Here's how the part is built. I have some questions about the finished solid (model axes, mm). Face numbers are marked on the shaded views. A direction names the side the tool comes from. Give positions to 0.01 mm unless a question says otherwise; leave off trailing zeros. Write each loop counter-clockwise with the first axis right and the second up, starting at its lowest first coordinate (ties: lowest second). Pieces come first, ordered by that corner, then holes. Notation, with made-up numbers: (70.25, 36.5) -> (79.25, 36.5) arc R14 cw to (79.25, 62.5) -> close; hole circle Ø7 at (89, 35). An arc over 180 degrees is marked (long way). Use one line per item in the form item = value.
```python
from build123d import *

# Parameters (mm, degrees)
F0_W     = 15
F0_H     = 9
F0_W_2   = 11
F0_H_2   = 5
F1_DEPTH = 4
F2_R     = 0.99999


# Not quite as in the source:
# - a fillet or chamfer is up to 0.001 mm smaller than in the source, because OpenCascade refuses the exact size


with BuildPart() as f1:
    # F0 (on Top) → F1 (new body)
    with BuildSketch(Plane.XY):
        with Locations((5.5, 2.5)):
            Rectangle(F0_W, F0_H)
        with Locations((5.5, 2.5)):
            Rectangle(F0_W_2, F0_H_2, mode=Mode.SUBTRACT)
    extrude(amount=F1_DEPTH)

    # F2 (radius 1 in the source; OpenCascade refuses exactly that, so slightly less here)
    f2_edges = [f1.edges().sort_by_distance(p)[0] for p in [
        (5.5, -2, 4),
        (13, 2.5, 4),
        (5.5, 0, 4),
        (-2, 2.5, 4),
        (0, 2.5, 4),
        (5.5, 7, 4),
        (5.5, 5, 4),
        (11, 2.5, 4),
        (-2, -2, 2),
        (13, -2, 2),
        (11, 0, 2),
        (0, 0, 2),
        (-2, 7, 2),
        (13, 7, 2),
        (11, 5, 2),
        (0, 5, 2),
    ]]
    fillet(f2_edges, radius=F2_R)


solid = f1.part
```
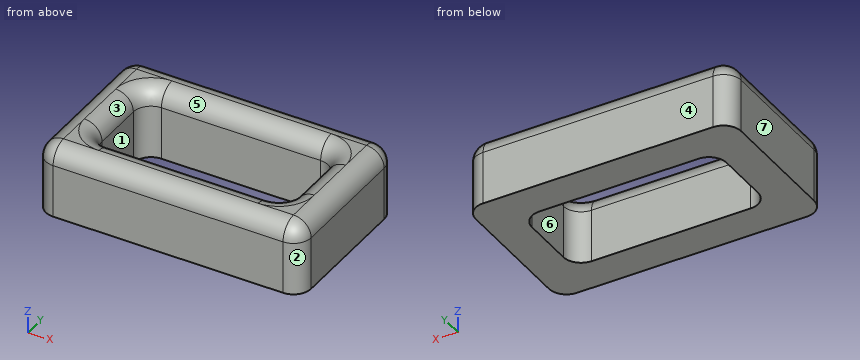
Q1. If I drill on line 1 along Y through (x, z) = (4.5, 1.1); line 2 along X through (y, z) = (4, 2.6); line 3 along X through (y, z) = (4.5, 2.3), over which ranges is the centre line in solid material (lowest first)? Write a range as from..to.
Result set:
line_1 = -2..0, 5..7
line_2 = -2..0, 11..13
line_3 = -2..0.13, 10.87..13
Q2. I want a section at C-C, the plane z = 1.7. Write out the boundary of the cut face in (x, y).
Result set:
outline = (-2, -1) arc R1 ccw to (-1, -2) -> (12, -2) arc R1 ccw to (13, -1) -> (13, 6) arc R1 ccw to (12, 7) -> (-1, 7) arc R1 ccw to (-2, 6) -> close; hole (0, 1) arc R1 ccw to (1, 0) -> (10, 0) arc R1 ccw to (11, 1) -> (11, 4) arc R1 ccw to (10, 5) -> (1, 5) arc R1 ccw to (0, 4) -> close
Q3. Which directions (+Z, -Z, +X, -X, +Y, -Y) give clear straight access to the entire face, cutting with the end or side of a thin tool? Please do the marked faces 1, 2 and 3.
Result set:
face_1 = +Z, -Z
face_2 = +Z, -Z, +X, -Y
face_3 = +Z
Q4. If we mould it in two halves opening along X, with no side actions, what happens to the marked faces 4, 5, 6 and 7? For each: +X half, -X half, draft (parallel to the pull), parting line (faces both ways), or undercut.
Result set:
face_4 = draft
face_5 = undercut
face_6 = undercut
face_7 = -X half
